Verification items for the finished model (mm, model axes). A direction names the side the tool comes from. Round coordinates to 2 decimals unless told otherwise and drop trailing zeros. Write each loop counter-clockwise with the first axis right and the second up, starting at its lowest first coordinate (ties: lowest second). Pieces come first, ordered by that corner, then holes. Notation, with made-up numbers: (67, 29) - (122, 29) arc R19 cw to (122, 53) - close; hole circle Ø2 at (69.25, 63). An arc over 180 degrees is marked (long way). Write each question's results on one line, items separated by ' | '.
```python
from build123d import *

# Parameters (mm, degrees)
SKETCH1_W           = 62
SKETCH1_H           = 54
BOSS_EXTRUDE1_DEPTH = 12
BOSS_EXTRUDE2_DEPTH = 52
SKETCH3_W           = 62
SKETCH3_H           = 54
BOSS_EXTRUDE3_DEPTH = 4
CUT_EXTRUDE1_DEPTH  = 7
SKETCH6_R           = 20
BOSS_EXTRUDE4_DEPTH = 6
SKETCH16_R          = 2
CUT_EXTRUDE3_DEPTH  = 11
SKETCH26_W          = 37
SKETCH26_H          = 4
CUT_EXTRUDE10_DEPTH = 48
SKETCH29_R          = 1
CUT_EXTRUDE12_DEPTH = 48
SKETCH31_R          = 12.5
BOSS_EXTRUDE7_DEPTH = 6
SKETCH33_R          = 6
SKETCH33_R_2        = 3
BOSS_EXTRUDE8_DEPTH = 12
SKETCH34_R          = 1
CUT_EXTRUDE13_DEPTH = 11
SKETCH35_R          = 2.5
CUT_EXTRUDE15_DEPTH = 3
SKETCH37_R          = 4
CUT_EXTRUDE16_DEPTH = 4
BOSS_EXTRUDE9_DEPTH = 10


with BuildPart() as part:
    # Sketch1 → Boss-Extrude1 (new body)
    with BuildSketch(Plane(origin=(0, 0, 0), x_dir=(1, 0, 0), z_dir=(0, 1, 0))):
        Rectangle(SKETCH1_W, SKETCH1_H)
    extrude(amount=BOSS_EXTRUDE1_DEPTH)

    # Sketch2 → Boss-Extrude2 (add)
    with BuildSketch(Plane(origin=(0, 12, 0), x_dir=(1, 0, 0), z_dir=(0, 1, 0))):
        Polygon((-31, -27), (-26, -27), (-26, 23), (26, 23), (26, -27), (31, -27), (31, 22.851296476), (31, 27), (-31, 27), (-31, 22.851296476), align=None)
    extrude(amount=BOSS_EXTRUDE2_DEPTH)

    # Sketch3 → Boss-Extrude3 (add)
    with BuildSketch(Plane(origin=(0, 64, 0), x_dir=(1, 0, 0), z_dir=(0, 1, 0))):
        Rectangle(SKETCH3_W, SKETCH3_H)
    extrude(amount=BOSS_EXTRUDE3_DEPTH)

    # Sketch9 → Ø20.0mm Dowel Hole1 (revolve, cut)
    with BuildSketch(Plane(origin=(0, 25, -23), x_dir=(0, -1, 0), z_dir=(1, 0, 0))):
        Polygon((0, 0), (0, 4), (10, 4), (10, 0.025), (10.025, 0), align=None)
    revolve(axis=Axis((0, 25, -16.65), (0, 0, -1)), mode=Mode.SUBTRACT)

    # Sketch14 → Cut-Extrude1 (cut)
    with BuildSketch(Plane(origin=(0, 12, 0), x_dir=(1, 0, 0), z_dir=(0, 1, 0))):
        with BuildLine():
            Line((-12, -9), (-12, -27))
            Line((-12, -27), (12, -27))
            Line((12, -27), (12, -9))
            ThreePointArc((12, -9), (0, 3), (-12, -9))
        make_face()
    extrude(amount=-CUT_EXTRUDE1_DEPTH, mode=Mode.SUBTRACT)

    # Sketch6 → Boss-Extrude4 (add)
    with BuildSketch(Plane.ZY.offset(31)):
        with Locations((0, 33)):
            Circle(SKETCH6_R)
    extrude(amount=BOSS_EXTRUDE4_DEPTH)

    # Sketch16 → Cut-Extrude3 (cut)
    with BuildSketch(Plane.ZY.offset(37)):
        with Locations((0, 49)):
            Circle(SKETCH16_R)
        with Locations((13.856406461, 41)):
            Circle(SKETCH16_R)
        with Locations((13.856406461, 25)):
            Circle(SKETCH16_R)
        with Locations((0, 17)):
            Circle(SKETCH16_R)
        with Locations((-13.856406461, 25)):
            Circle(SKETCH16_R)
        with Locations((-13.856406461, 41)):
            Circle(SKETCH16_R)
    extrude(amount=-CUT_EXTRUDE3_DEPTH, mode=Mode.SUBTRACT)

    # Sketch26 → Cut-Extrude10 (cut)
    with BuildSketch(Plane.XY.offset(27)):
        with Locations((0, 66)):
            Rectangle(SKETCH26_W, SKETCH26_H)
    extrude(amount=-CUT_EXTRUDE10_DEPTH, mode=Mode.SUBTRACT)

    # Sketch29 → Cut-Extrude12 (cut)
    with BuildSketch(Plane(origin=(0, 5, 0), x_dir=(1, 0, 0), z_dir=(0, 1, 0))):
        with Locations(Location((0, -8.367265469, 0), (0, 0, 270))):
            Circle(SKETCH29_R)
    extrude(amount=-CUT_EXTRUDE12_DEPTH, mode=Mode.SUBTRACT)

    # Sketch31 → Boss-Extrude7 (add)
    with BuildSketch(Plane(origin=(31, 0, 0), x_dir=(0, 0, -1), z_dir=(1, 0, 0))):
        with Locations((0, 33)):
            Circle(SKETCH31_R)
    extrude(amount=BOSS_EXTRUDE7_DEPTH)

    # Sketch33 → Boss-Extrude8 (add)
    with BuildSketch(Plane(origin=(37, 0, 0), x_dir=(0, 0, -1), z_dir=(1, 0, 0))):
        with Locations((0, 33)):
            Circle(SKETCH33_R)
        with Locations((0, 33)):
            Circle(SKETCH33_R_2, mode=Mode.SUBTRACT)
    extrude(amount=BOSS_EXTRUDE8_DEPTH)

    # Sketch34 → Cut-Extrude13 (cut)
    with BuildSketch(Plane.ZY.offset(37)):
        with Locations((-4.949747468, 37.949747468)):
            Circle(SKETCH34_R)
        with Locations((4.949747468, 37.949747468)):
            Circle(SKETCH34_R)
        with Locations((4.949747468, 28.050252532)):
            Circle(SKETCH34_R)
        with Locations((-4.949747468, 28.050252532)):
            Circle(SKETCH34_R)
    extrude(amount=-CUT_EXTRUDE13_DEPTH, mode=Mode.SUBTRACT)

    # Sketch35 → Cut-Extrude15 (cut)
    with BuildSketch(Plane(origin=(-26, 0, 0), x_dir=(0, 0, -1), z_dir=(1, 0, 0))):
        with Locations((-4.949747468, 37.949747468)):
            Circle(SKETCH35_R)
        with Locations((4.949747468, 37.949747468)):
            Circle(SKETCH35_R)
        with Locations((4.949747468, 28.050252532)):
            Circle(SKETCH35_R)
        with Locations((-4.949747468, 28.050252532)):
            Circle(SKETCH35_R)
    extrude(amount=-CUT_EXTRUDE15_DEPTH, mode=Mode.SUBTRACT)

    # Sketch37 → Cut-Extrude16 (cut)
    with BuildSketch(Plane(origin=(-26, 0, 0), x_dir=(0, 0, -1), z_dir=(1, 0, 0))):
        with Locations((0, 49)):
            Circle(SKETCH37_R)
        with Locations((13.856406461, 41)):
            Circle(SKETCH37_R)
        with Locations((13.856406461, 25)):
            Circle(SKETCH37_R)
        with Locations((0, 17)):
            Circle(SKETCH37_R)
        with Locations((-13.856406461, 25)):
            Circle(SKETCH37_R)
        with Locations((-13.856406461, 41)):
            Circle(SKETCH37_R)
    extrude(amount=-CUT_EXTRUDE16_DEPTH, mode=Mode.SUBTRACT)

    # Sketch38 → Boss-Extrude9 (add)
    with BuildSketch(Plane(origin=(37, 0, 0), x_dir=(0, 0, -1), z_dir=(1, 0, 0))):
        with BuildLine():
            Line((1.658312395, 35.5), (-1.658312395, 35.5))
            ThreePointArc((-1.658312395, 35.5), (0, 36), (1.658312395, 35.5))
        make_face()
    extrude(amount=BOSS_EXTRUDE9_DEPTH)


solid = part.part
```
(1) Go/stop test with flat-tipped pins: pin 1 Ø20 at (y, z) = (27, -2.5) entering from +X; pin 2 Ø3.5 at (y, z) = (41, 13.86) entering from +X; pin 3 Ø12 at (x, z) = (4.5, 15.5) entering from +Y; pin 4 Ø3 at (x, z) = (37, 0.5) entering from +Y. Record where each tip stops, or that it passes through.
Answer:
pin 1: x = 49 | pin 2: x = 31 | pin 3: y = 5 | pin 4: y = 45.5
(2) Section check C-C (y = 62). Record the cut outline in (x, z).
Answer:
outline: (-31, -27) - (31, -27) - (31, 27) - (26, 27) - (26, -23) - (-26, -23) - (-26, 27) - (-31, 27) - close
(3) Mould release check, pull along Z, two halves, no side actions. Record for faces 1 (the flat face through (14, 11, 27)), 2 (the flat face through (0, 0, 0)), 3 (the cylindrical face through (-34, 19, 0)), 4 (the cylindrical face through (-33.056, 36.974, 4.733)): released by +Z, released by -Z, zero draft, split by the parting line, or undercut.
Answer:
face 1: released by +Z | face 2: zero draft | face 3: undercut | face 4: undercut
(4) Thickness scan on L1, parallel to Y at x = -33.75, z = 0; L2, parallel to X at y = 33, z = 21; L3, parallel to X at y = 45, z = 9.5. Record the ranges inside material, lowest first.
Answer:
L1: 13 to 15, 19 to 47, 51 to 53 | L2: -31 to -26, 26 to 31 | L3: -37 to -26, 26 to 31
(5) Set-up check for faces 5 (the cylindrical face through (-33.06, 27.44, -5.74)), 6 (the flat face through (0, 66, -21)), 7 (the flat face through (-29, 37, -6)), 8 (the flat face through (0, 12, -4)): record each of +Z, -Z, +X, -X, +Y, -Y from which the full face is reachable in a straight line by a thin tool's end or side.
Answer:
face 5: -X | face 6: +Z, +Y | face 7: none | face 8: +Z
(6) Section check B-B (y = 49). Record the cut outline in (x, z), plus the area to 3 significant figures.
Answer:
outline: (-37, -12) - (-31, -12) - (-31, -27) - (31, -27) - (31, 27) - (26, 27) - (26, -23) - (-26, -23) - (-26, -4) - (-30, -4) - (-30, -2) - (-37, -2) - close; (-37, 2) - (-30, 2) - (-30, 4) - (-26, 4) - (-26, 27) - (-31, 27) - (-31, 12) - (-37, 12) - close | area: 832 mm2
(7) Section check A-A (x = 0). Record the cut outline in (y, z) (3 decimals).
Answer:
outline: (0, -27) - (15, -27) - (15, -23.025) - (14.975, -23) - (12, -23) - (12, -3) - (5, -3) - (5, 7.367) - (0, 7.367) - close; (0, 9.367) - (5, 9.367) - (5, 27) - (0, 27) - close; (35, -27) - (68, -27) - (68, -21) - (64, -21) - (64, -23) - (35.025, -23) - (35, -23.025) - close
(8) Section check D-D (x = -13). Record the cut outline in (y, z).
Answer:
outline: (0, -27) - (68, -27) - (68, -21) - (64, -21) - (64, -23) - (12, -23) - (12, 27) - (0, 27) - close
